```python
from build123d import *

# Parameters (mm, degrees)
BOSS_EXTRUDE1_DEPTH = 5
CUT_EXTRUDE1_REACH  = 41.083
CUT_EXTRUDE2_REACH  = 41.364
FILLET1_R           = 1


with BuildPart() as part:
    # Sketch1 → Boss-Extrude1 (new body)
    with BuildSketch(Plane(origin=(0, 0, 0), x_dir=(1, 0, 0), z_dir=(0, 1, 0))):
        with BuildLine():
            Line((-33.99999999999999, 2), (-33.99999999999999, -2))
            Line((-33.99999999999999, -2), (-29.968871125850622, -2))
            ThreePointArc((-29.968871125850665, -1.9999999999998734), (-29.618785560277153, -1.0271124734730797), (-29.5, -1.1e-15))
            ThreePointArc((-29.5, 0), (-29.618785560277153, 1.0271124734730805), (-29.968871125850665, 1.9999999999998725))
            Line((-29.968871125850622, 2), (-33.99999999999999, 2))
        make_face()
        with BuildLine():
            Line((-29.968871125850622, -2), (-33.99999999999999, -2))
            Line((-33.99999999999999, -2), (-33.99999999999999, 2))
            Line((-33.99999999999999, 2), (-29.968871125850622, 2))
            ThreePointArc((-29.968871125850665, 1.9999999999998725), (-38.499999999999986, 5.5e-16), (-29.968871125850665, -1.9999999999998734))
        make_face()
        with BuildLine():
            ThreePointArc((-29.5, -1.1e-15), (-29.618785560277153, -1.0271124734730797), (-29.968871125850665, -1.9999999999998734))
            Line((-29.968871125850622, -2), (29.96887112585072, -2))
            ThreePointArc((29.96887112585073, -1.9999999999999722), (29.500000000000014, 5.5e-16), (29.96887112585073, 1.9999999999999731))
            Line((29.96887112585072, 2), (-29.968871125850622, 2))
            ThreePointArc((-29.968871125850665, 1.9999999999998725), (-29.618785560277153, 1.0271124734730805), (-29.5, 0))
        make_face()
        with BuildLine():
            ThreePointArc((29.96887112585073, 1.9999999999999731), (29.500000000000014, 5.5e-16), (29.96887112585073, -1.9999999999999722))
            Line((29.96887112585072, -2), (34.00000000000001, -2))
            Line((34.00000000000001, -2), (34.00000000000001, 2))
            Line((34.00000000000001, 2), (29.96887112585072, 2))
        make_face()
        with BuildLine():
            Line((34.00000000000001, -2), (29.96887112585072, -2))
            ThreePointArc((29.96887112585073, -1.9999999999999722), (35.02711247347314, -4.38121443972283), (38.5, -1.1e-15))
            ThreePointArc((38.5, 0), (35.02711247347314, 4.381214439722829), (29.96887112585073, 1.9999999999999731))
            Line((29.96887112585072, 2), (34.00000000000001, 2))
            Line((34.00000000000001, 2), (34.00000000000001, -2))
        make_face()
    extrude(amount=BOSS_EXTRUDE1_DEPTH)

    # Cut-Sweep1: sweep along a path in Sketch2
    with BuildLine(Plane(origin=(0, 5, 0), x_dir=(1, 0, 0), z_dir=(0, 1, 0))) as cut_sweep1_path:
        CenterArc((-33.99999999999999, 0), 4.499999999999991, 0, 360)
    # 3DSketch1 → Cut-Sweep1 (sweep, cut)
    with BuildSketch(Plane(origin=(-33.99999999999999, 5, 0), x_dir=(0, -1, 0), z_dir=(-1, 0, 0))):
        with BuildLine():
            Line((0, 0), (-1.5000000000000004, 0))
            ThreePointArc((-1.5000000000000004, 0), (1.25, 2.75), (4, 0))
            Line((4, 0), (0, 0))
        make_face()
    cut_sweep1 = sweep(path=cut_sweep1_path.line, mode=Mode.SUBTRACT)

    # Mirror1: Cut-Sweep1 across plane
    add(cut_sweep1.mirror(Plane(origin=(0, 0, 0), x_dir=(0, 0, 1), z_dir=(1, 0, 0))), mode=Mode.SUBTRACT)

    # Cut-Extrude1: up to this face of the body (flat: up to its plane)
    cut_extrude1_end = Plane(part.part.faces().sort_by_distance((0, 5, -2.639e-06))[0])
    # Sketch3 → Cut-Extrude1 (cut, up to the picked face)
    with BuildSketch(Plane.XZ, mode=Mode.PRIVATE) as cut_extrude1_sk1:
        with BuildLine():
            ThreePointArc((-29.52786404500042, 0.49999999999997785), (-29.506971411314076, 0.2503879015666308), (-29.5, 0))
            Line((-29.5, 0), (-23.999999999999993, 0))
            Line((-23.999999999999993, 0), (-23.999999999999993, 0.5))
            Line((-23.999999999999993, 0.5), (-29.527864045000417, 0.5))
        make_face()
    cut_extrude1_tool1 = split(extrude(cut_extrude1_sk1.sketch, amount=-CUT_EXTRUDE1_REACH, mode=Mode.PRIVATE), bisect_by=cut_extrude1_end, keep=Keep.BOTH, mode=Mode.PRIVATE)
    # Sketch3 → Cut-Extrude1 (cut, up to the picked face)
    with BuildSketch(Plane.XZ, mode=Mode.PRIVATE) as cut_extrude1_sk2:
        with BuildLine():
            Line((-23.999999999999993, 0), (-29.5, 0))
            ThreePointArc((-29.5, -1.1e-15), (-29.506971411314076, -0.25038790156662954), (-29.52786404500042, -0.49999999999997824))
            Line((-29.527864045000417, -0.5), (-23.999999999999993, -0.5))
            Line((-23.999999999999993, -0.5), (-23.999999999999993, 0))
        make_face()
    cut_extrude1_tool2 = split(extrude(cut_extrude1_sk2.sketch, amount=-CUT_EXTRUDE1_REACH, mode=Mode.PRIVATE), bisect_by=cut_extrude1_end, keep=Keep.BOTH, mode=Mode.PRIVATE)
    # Sketch3 → Cut-Extrude1 (cut, up to the picked face)
    with BuildSketch(Plane.XZ, mode=Mode.PRIVATE) as cut_extrude1_sk3:
        with BuildLine():
            Line((-33.99999999999999, 0.5), (-33.99999999999999, 0))
            Line((-33.99999999999999, 0), (-29.5, 0))
            ThreePointArc((-29.5, 0), (-29.506971411314076, 0.2503879015666308), (-29.52786404500042, 0.49999999999997785))
            Line((-29.527864045000417, 0.5), (-33.99999999999999, 0.5))
        make_face()
    cut_extrude1_tool3 = split(extrude(cut_extrude1_sk3.sketch, amount=-CUT_EXTRUDE1_REACH, mode=Mode.PRIVATE), bisect_by=cut_extrude1_end, keep=Keep.BOTH, mode=Mode.PRIVATE)
    # Sketch3 → Cut-Extrude1 (cut, up to the picked face)
    with BuildSketch(Plane.XZ, mode=Mode.PRIVATE) as cut_extrude1_sk4:
        with BuildLine():
            Line((-29.5, 0), (-33.99999999999999, 0))
            Line((-33.99999999999999, 0), (-33.99999999999999, -0.5))
            Line((-33.99999999999999, -0.5), (-29.527864045000417, -0.5))
            ThreePointArc((-29.52786404500042, -0.49999999999997824), (-29.506971411314076, -0.25038790156662954), (-29.5, -1.1e-15))
        make_face()
    cut_extrude1_tool4 = split(extrude(cut_extrude1_sk4.sketch, amount=-CUT_EXTRUDE1_REACH, mode=Mode.PRIVATE), bisect_by=cut_extrude1_end, keep=Keep.BOTH, mode=Mode.PRIVATE)
    cut_extrude1_1 = cut_extrude1_tool1.solids().sort_by(Axis((-26.754644, 0, 0.250211), (0, 1, 0)))[0]
    add(cut_extrude1_1, mode=Mode.SUBTRACT)
    cut_extrude1_2 = cut_extrude1_tool2.solids().sort_by(Axis((-26.754644, 0, -0.250211), (0, 1, 0)))[0]
    add(cut_extrude1_2, mode=Mode.SUBTRACT)
    cut_extrude1_3 = cut_extrude1_tool3.solids().sort_by(Axis((-31.754631, 0, 0.249742), (0, 1, 0)))[0]
    add(cut_extrude1_3, mode=Mode.SUBTRACT)
    cut_extrude1_4 = cut_extrude1_tool4.solids().sort_by(Axis((-31.754631, 0, -0.249742), (0, 1, 0)))[0]
    add(cut_extrude1_4, mode=Mode.SUBTRACT)
    cut_extrude1 = cut_extrude1_1 + cut_extrude1_2 + cut_extrude1_3 + cut_extrude1_4  # Cut-Extrude1 as one shape, for the pattern or mirror that repeats it

    # Mirror2: Cut-Extrude1 across plane
    add(cut_extrude1.mirror(Plane(origin=(0, 0, 0), x_dir=(0, 0, 1), z_dir=(1, 0, 0))), mode=Mode.SUBTRACT)

    # Cut-Extrude2: up to this face of the body (flat: up to its plane)
    cut_extrude2_end = Plane(part.part.faces().sort_by_distance((0, 2.5, 2))[0])
    # Sketch4 → Cut-Extrude2 (cut, up to the picked face)
    with BuildSketch(Plane(origin=(0, 0, -2), x_dir=(-1, 0, 0), z_dir=(0, 0, -1)), mode=Mode.PRIVATE) as cut_extrude2_sk1:
        Polygon((23.99999999999999, 1.5000000000000009), (28.178209788095508, 1.5000000000000009), (25.790661337755214, 3.5000000000000004), (23.99999999999999, 3.500000000000001), align=None)
    cut_extrude2_tool1 = split(extrude(cut_extrude2_sk1.sketch, amount=-CUT_EXTRUDE2_REACH, mode=Mode.PRIVATE), bisect_by=cut_extrude2_end, keep=Keep.BOTH, mode=Mode.PRIVATE)
    # Sketch4 → Cut-Extrude2 (cut, up to the picked face)
    with BuildSketch(Plane(origin=(0, 0, -2), x_dir=(-1, 0, 0), z_dir=(0, 0, -1)), mode=Mode.PRIVATE) as cut_extrude2_sk2:
        Polygon((25.790661337755214, 3.5000000000000004), (28.178209788095508, 1.5000000000000007), (29.96887112585073, 1.5000000000000009), (29.96887112585073, 3.500000000000001), align=None)
    cut_extrude2_tool2 = split(extrude(cut_extrude2_sk2.sketch, amount=-CUT_EXTRUDE2_REACH, mode=Mode.PRIVATE), bisect_by=cut_extrude2_end, keep=Keep.BOTH, mode=Mode.PRIVATE)
    cut_extrude2_1 = cut_extrude2_tool1.solids().sort_by(Axis((-25.571803, 2.366667, -2), (0, 0, 1)))[0]
    add(cut_extrude2_1, mode=Mode.SUBTRACT)
    cut_extrude2_2 = cut_extrude2_tool2.solids().sort_by(Axis((-28.397068, 2.633333, -2), (0, 0, 1)))[0]
    add(cut_extrude2_2, mode=Mode.SUBTRACT)
    cut_extrude2 = cut_extrude2_1 + cut_extrude2_2  # Cut-Extrude2 as one shape, for the pattern or mirror that repeats it

    # Mirror3: Cut-Extrude2 across plane
    add(cut_extrude2.mirror(Plane(origin=(0, 0, 0), x_dir=(0, 0, 1), z_dir=(1, 0, 0))), mode=Mode.SUBTRACT)

    # Fillet1
    fillet1_edges = [part.edges().sort_by_distance(p)[0] for p in [
        (3.908e-14, 5, 1.9999999999999665),
        (38.5, 5, 4.44e-15),
        (3.553e-14, 5, -1.999999999999966),
        (-38.50000000000023, 5, 5.89e-14),
        (3.553e-14, 0, -1.999999999999966),
        (38.5, 0, -2e-15),
        (3.908e-14, 0, 1.9999999999999665),
        (-38.50000000000024, 0, -6.573e-14),
    ]]
    fillet(fillet1_edges, radius=FILLET1_R)


solid = part.part
```
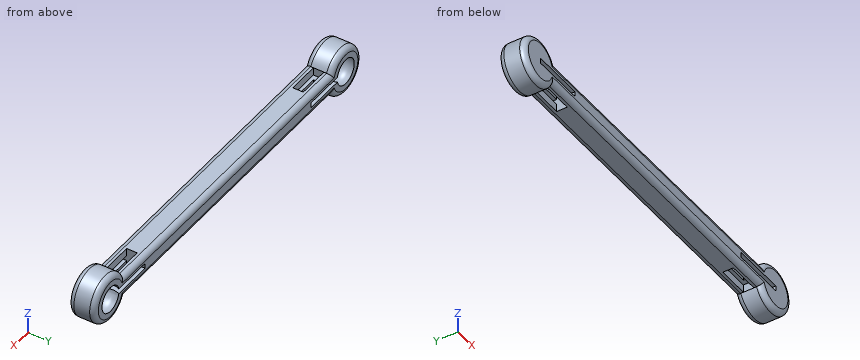
Work out the finished part from the listing and answer in its coordinate system (mm). Coordinates: 2 decimals unless noted, no trailing zeros. Order: outer loops, then holes, each group sorted by start corner. A loop starts at its lowest first (then second) coordinate and runs counter-clockwise, first axis right, second up. Notation, with made-up numbers: (-28.75, 73) - (7.25, 73) arc R31 ccw to (7.25, 106) - close; hole circle Ø1 at (-33, -30.75). An arc over 180 degrees is marked (long way). Answer as a JSON object with one key per item and string values.
1. Consider line 1 (X direction, y = 2.5, z = 0.25); line 2 (X direction, y = 1.75, z = 1); line 3 (Z direction, x = 26, y = 4.65). Determine where each line is inside the solid, lowest interval first.
Output values:
{"line 1": "x = -38.49 to -36.44, -24 to 24, 36.44 to 38.49", "line 2": "x = -38.39 to -35.6, -32.4 to -29.97, -24 to 24, 29.97 to 32.4, 35.6 to 38.39", "line 3": "z = -1.76 to -0.5, 0.5 to 1.76"}
2. Find section B-B on x = -10. Determine the outline of the cut face in (y, z).
Output values:
{"outline": "(0, -1) arc R1 ccw to (1, -2) - (4, -2) arc R1 ccw to (5, -1) - (5, 1) arc R1 ccw to (4, 2) - (1, 2) arc R1 ccw to (0, 1) - close"}
3. Each of these flat-tipped pins is pushed along its axis until it touches: P1, Ø0.5, axis at y = 0.5, z = 0, coming from the -X side; P2, Ø1.5, axis at y = 3.5, z = 2.5, coming from the -X side; P3, Ø2.5, axis at x = 29, y = 2, coming from the -Z side. Where does it stop, or does it pass through?
Output values:
{"P1": "stops at x = -38.47", "P2": "stops at x = -38.15", "P3": "stops at z = -2.49"}
4. Find section A-A on x = 27. Determine the outline of the cut face in (y, z).
Output values:
{"outline": "(0, -1) arc R1 ccw to (1, -2) - (1.5, -2) - (1.5, -0.5) - (0, -0.5) - close; (0, 0.5) - (1.5, 0.5) - (1.5, 2) - (1, 2) arc R1 ccw to (0, 1) - close; (3.5, -2) - (4, -2) arc R1 ccw to (5, -1) - (5, -0.5) - (3.5, -0.5) - close; (3.5, 0.5) - (5, 0.5) - (5, 1) arc R1 ccw to (4, 2) - (3.5, 2) - close"}
